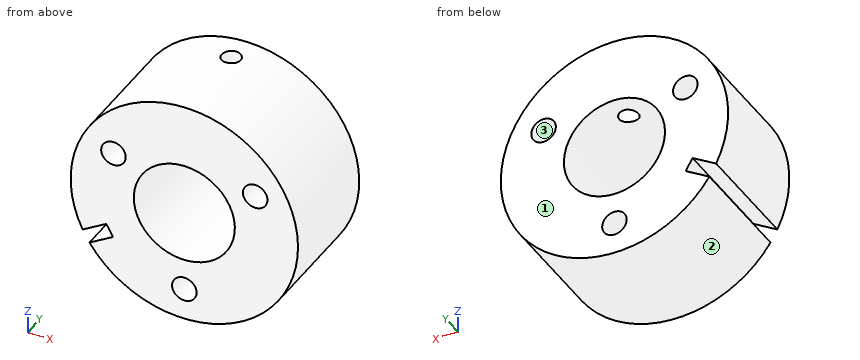
```python
from build123d import *

# Parameters (mm, degrees)
SKETCH1_R                  = 11.1125
SKETCH1_R_2                = 2.7
BOSS_EXTRUDE1_DEPTH        = 12.7
M5X0_8_TAPPED_HOLE1_REACH  = 61.172
M5X0_8_TAPPED_HOLE1_BORE_R = 2.1


with BuildPart() as part:
    # Sketch1 → Boss-Extrude1 (new, symmetric)
    with BuildSketch(Plane(origin=(0, 0, 0), x_dir=(1, 0, 0), z_dir=(0, 1, 0))):
        with BuildLine():
            Line((-15.665476391, 10.776517819), (-20.861628814, 13.776517819))
            ThreePointArc((-20.861628814, 13.776517819), (21.650635095, -12.5), (-22.361628814, 11.178441608))
            Line((-22.361628814, 11.178441608), (-17.165476391, 8.178441608))
            Line((-17.165476391, 8.178441608), (-15.665476391, 10.776517819))
        make_face()
        with Locations(Location((0, 0, 0), (0, 0, 270))):
            Circle(SKETCH1_R, mode=Mode.SUBTRACT)
        with Locations(Location((0, 18, 0), (0, 0, 270))):
            Circle(SKETCH1_R_2, mode=Mode.SUBTRACT)
        with Locations(Location((15.588457268, -9, 0), (0, 0, 270))):
            Circle(SKETCH1_R_2, mode=Mode.SUBTRACT)
        with Locations(Location((-15.588457268, -9, 0), (0, 0, 270))):
            Circle(SKETCH1_R_2, mode=Mode.SUBTRACT)
    extrude(amount=BOSS_EXTRUDE1_DEPTH, both=True)

    # M5x0.8 Tapped Hole1 bore (on position points) → M5x0.8 Tapped Hole1 (cut, up to next)
    with BuildSketch(Plane(origin=(0, 6.7, 25), x_dir=(1, 0, 0), z_dir=(0, 0, 1)), mode=Mode.PRIVATE) as m5x0_8_tapped_hole1_sk1:
        Circle(M5X0_8_TAPPED_HOLE1_BORE_R)
    m5x0_8_tapped_hole1_tool1 = extrude(m5x0_8_tapped_hole1_sk1.sketch, amount=-M5X0_8_TAPPED_HOLE1_REACH, mode=Mode.PRIVATE) & part.part
    add(m5x0_8_tapped_hole1_tool1.solids().sort_by_distance((0, 6.7, 25))[0], mode=Mode.SUBTRACT)


solid = part.part
```
Geometry check sheet. Reference: the model listing, model coordinates, mm. Face numbers are marked on the shaded views. Coordinates: 2 decimals unless noted, no trailing zeros. Loops run counter-clockwise (first coordinate to the right, second up) from the corner with the lowest first, then second, coordinate; pieces in that order, holes last.
Item 1: Sectioned sample at D-D, the plane z = 12.5. Record the boundary of the cut face in (x, y).
Item 2: Sectioned sample at C-C, the plane y = -5. Record the boundary of the cut face in (x, z) (1 decimal), then the cut area to 3 significant figures.
Item 3: Go/stop test with flat-tipped pins: pin 1 Ø2 at (x, y) = (17.5, 1.5) entering from -Z; pin 2 Ø12 at (y, z) = (5.5, -12.5) entering from +X; pin 3 Ø1.5 at (y, z) = (-7, 9.5) entering from +X; pin 4 Ø7 at (x, z) = (15.59, 9) entering from +Y. Record where each tip stops, or that it passes through.
Item 4: Thickness scan on line 1 (Y direction, x = 0, z = 15); line 2 (X direction, y = 5.5, z = 8); line 3 (X direction, y = 1.75, z = 0). Record the ranges inside material, lowest first.
Item 5: Release check for a two-part mould opening along Z. For the marked faces 1, 2 and 3 record: released by +Z, released by -Z, zero draft, split by the parting line, or undercut.
Item 6: Sectioned sample at A-A, the plane z = 0. Record the boundary of the cut face in (x, y).
Item 7: Sectioned sample at B-B, the plane x = 0. Record the boundary of the cut face in (y, z).
Check result:
1. outline: (-21.65, -12.7) - (21.65, -12.7) - (21.65, 12.7) - (-21.65, 12.7) - close; hole circle Ø4.2 at (0, 6.7)
2. outline: (-22.4, -11.2) - (-17.2, -8.2) - (-15.7, -10.8) - (-20.9, -13.8) arc R25 ccw (long way) to start; hole circle Ø5.4 at (-15.6, 9); hole circle Ø22.2 at (0, 0); hole circle Ø5.4 at (0, -18); hole circle Ø5.4 at (15.6, 9)
2. area: 1,490 mm2
3. pin 1: stops at z = -18.78
3. pin 2: stops at x = 24.14
3. pin 3: stops at x = 23.42
3. pin 4: stops at y = 12.7
4. line 1: y = -12.7 to 4.6, 8.8 to 12.7
4. line 2: x = -23.69 to -18.1, -13.08 to -7.71, 7.71 to 13.08, 18.1 to 23.69
4. line 3: x = -25 to -11.11, 11.11 to 25
5. face 1: zero draft
5. face 2: split by the parting line
5. face 3: undercut
6. outline: (-25, -12.7) - (-11.11, -12.7) - (-11.11, 12.7) - (-25, 12.7) - close; (11.11, -12.7) - (25, -12.7) - (25, 12.7) - (11.11, 12.7) - close
7. outline: (-12.7, -25) - (12.7, -25) - (12.7, -20.7) - (-12.7, -20.7) - close; (-12.7, -15.3) - (12.7, -15.3) - (12.7, -11.11) - (-12.7, -11.11) - close; (-12.7, 11.11) - (4.6, 11.11) - (4.6, 25) - (-12.7, 25) - close; (8.8, 11.11) - (12.7, 11.11) - (12.7, 25) - (8.8, 25) - close
